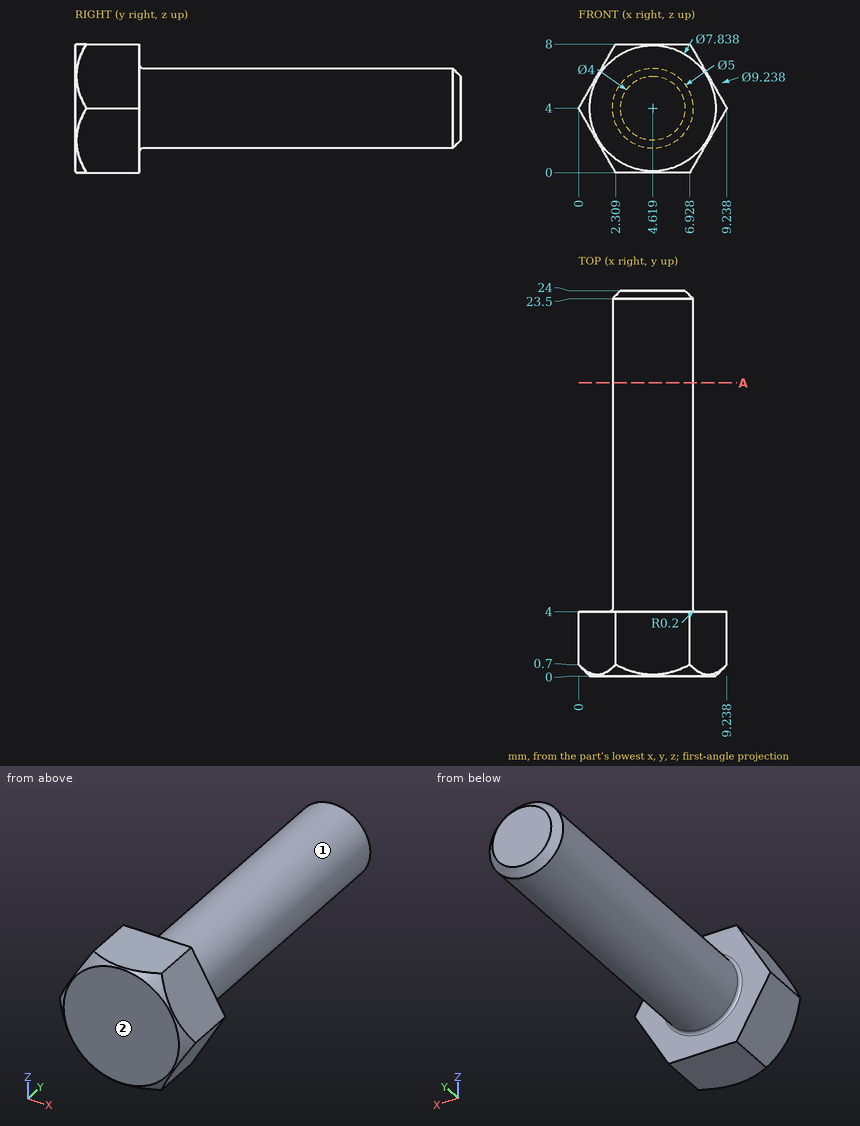
Geometry: see drawing. Coordinates: mm, zero at the bounding-box minimum. A direction names the side the tool comes from. Round coordinates to 2 decimals unless told otherwise and drop trailing zeros. Loops run counter-clockwise (first coordinate to the right, second up) from the corner with the lowest first, then second, coordinate; pieces in that order, holes last. Notation, with made-up numbers: (4, 68) -> (55, 68) arc R18 ccw to (55, 95) -> close; hole circle Ø2 at (-3.75, 43). An arc over 180 degrees is marked (long way). One line per question, with ' | ' between items. Start each with the question number.
1. Section A-A on y = 18.25. Output: boundary loops of the cut face in (x, z), and give its area (3 significant figures).
2. Line query: line 1 along Y through (x, z) = (3, 0.75); line 2 along X through (y, z) = (13.5, 5.5); line 3 along X through (y, z) = (20.5, 5.75) (1 decimal). Output: solid intervals per line, ascending. Write a range as [from, to].
3. Set-up query: the marked faces 1 and 2. Return all of +Z, -Z, +X, -X, +Y, -Y with unobstructed straight access to the full face (end or side cutting, diameter ignored); none if empty.
4. Contact query for flat-ended pins moving along their axis: pin 1 (3 mm diameter, centred on x = 5.5, z = 4.5, fed in from -Y); pin 2 (4 mm diameter, centred on x = 3.5, y = 16.5, fed in from -Z); pin 3 (1 mm diameter, centred on x = 2.5, z = 1.5, fed in from +Y); pin 4 (1.5 mm diameter, centred on y = 5, z = 6, fed in from +X). Output: stop coordinate, or through.
Returned:
1) outline: circle Ø5 at (4.62, 4) | area: 19.6 mm2
2) line 1: y = [0, 4] | line 2: x = [2.62, 6.62] | line 3: x = [2.8, 6.4]
3) face 1: +Y | face 2: +Z, -Z, +X, -X, -Y
4) pin 1: stops at y = 0 | pin 2: stops at z = 1.5 | pin 3: stops at y = 4 | pin 4: stops at x = 6.78
